from build123d import *

# Parameters (mm, degrees)
SKETCH_W     = 80
SKETCH_H     = 26
PAD_DEPTH    = 2
SKETCH001_W  = 73.5
SKETCH001_H  = 21.5
PAD001_DEPTH = 2
SKETCH002_W  = 1.5
SKETCH002_H  = 20
POCKET_DEPTH = 5
CHAMFER_SIZE = 1.5


with BuildPart() as part:
    # Sketch → Pad (new body)
    with BuildSketch(Plane.XY):
        Rectangle(SKETCH_W, SKETCH_H)
    extrude(amount=PAD_DEPTH)

    # Sketch001 (on Face6 of Pad) → Pad001 (join)
    with BuildSketch(Plane.XY.offset(2)):
        Rectangle(SKETCH001_W, SKETCH001_H)
    extrude(amount=PAD001_DEPTH)

    # Sketch002 (on Face11 of Pad001) → Pocket (cut)
    with BuildSketch(Plane.XY.offset(4)):
        with Locations((1.5, 0)):
            Rectangle(SKETCH002_W, SKETCH002_H)
        with Locations((4.5, 0)):
            Rectangle(SKETCH002_W, SKETCH002_H)
        with Locations((7.5, 0)):
            Rectangle(SKETCH002_W, SKETCH002_H)
        with Locations((10.5, 0)):
            Rectangle(SKETCH002_W, SKETCH002_H)
        with Locations((13.5, 0)):
            Rectangle(SKETCH002_W, SKETCH002_H)
        with Locations((16.5, 0)):
            Rectangle(SKETCH002_W, SKETCH002_H)
        with Locations((19.5, 0)):
            Rectangle(SKETCH002_W, SKETCH002_H)
        with Locations((22.5, 0)):
            Rectangle(SKETCH002_W, SKETCH002_H)
        with Locations((25.5, 0)):
            Rectangle(SKETCH002_W, SKETCH002_H)
        with Locations((28.5, 0)):
            Rectangle(SKETCH002_W, SKETCH002_H)
        with Locations((31.5, 0)):
            Rectangle(SKETCH002_W, SKETCH002_H)
        with Locations((34.5, 0)):
            Rectangle(SKETCH002_W, SKETCH002_H)
        with Locations((-1.5, 0)):
            Rectangle(SKETCH002_W, SKETCH002_H)
        with Locations((-4.5, 0)):
            Rectangle(SKETCH002_W, SKETCH002_H)
        with Locations((-7.5, 0)):
            Rectangle(SKETCH002_W, SKETCH002_H)
        with Locations((-10.5, 0)):
            Rectangle(SKETCH002_W, SKETCH002_H)
        with Locations((-13.5, 0)):
            Rectangle(SKETCH002_W, SKETCH002_H)
        with Locations((-16.5, 0)):
            Rectangle(SKETCH002_W, SKETCH002_H)
        with Locations((-19.5, 0)):
            Rectangle(SKETCH002_W, SKETCH002_H)
        with Locations((-22.5, 0)):
            Rectangle(SKETCH002_W, SKETCH002_H)
        with Locations((-25.5, 0)):
            Rectangle(SKETCH002_W, SKETCH002_H)
        with Locations((-28.5, 0)):
            Rectangle(SKETCH002_W, SKETCH002_H)
        with Locations((-31.5, 0)):
            Rectangle(SKETCH002_W, SKETCH002_H)
        with Locations((-34.5, 0)):
            Rectangle(SKETCH002_W, SKETCH002_H)
    extrude(amount=-POCKET_DEPTH, mode=Mode.SUBTRACT)

    # Chamfer
    chamfer_edges = [part.edges().sort_by_distance(p)[0] for p in [
        (0, -13, 0),
        (40, 0, 0),
        (0, 13, 0),
        (-40, 0, 0),
    ]]
    chamfer(chamfer_edges, length=CHAMFER_SIZE)


solid = part.part
Model file for the job. Use its own axes, mm. Give positions to 0.01 mm unless a question says otherwise; leave off trailing zeros. Loops run counter-clockwise (first coordinate to the right, second up) from the corner with the lowest first, then second, coordinate; pieces in that order, holes last.
1) Saw through at B-B (y = 8.25). Count the separate pieces of the cut face and the enclosed holes in it, plus the area to 3 significant figures.
2) Saw through at A-A (x = -19.5). Write the cut outline in (y, z).
3) Pull direction Y, two halves, no side cores. Call faces 1 (the flat face through (36.75, 0, 3)), 2 (the flat face through (18.75, 0, 2)), 3 (the flat face through (-0.6, -12.2, 0.7)): +Y half, -Y half, draft (parallel to the pull), parting line (faces both ways), or undercut.
4) Wall check: line 1 (Y direction, x = 13.5, z = 1.7); line 2 (Y direction, x = 25, z = 3); line 3 (Y direction, x = -15, z = 3.1). Give the ranges that are in metal, low to high.
5) Flat gauge pins, fed straight in: pin 1 Ø0.8 at (x, z) = (-13.5, 3) entering from -Y; pin 2 Ø6 at (x, y) = (-18, -2.5) entering from -Z. Where does each tip first touch, or does it go through?
Answer block:
1. separate pieces: 25
1. enclosed holes: 0
1. area: 161 mm2
2. outline: (-13, 1.5) - (-11.5, 0) - (-10, 0) - (-10, 4) - (-10.75, 4) - (-10.75, 2) - (-13, 2) - close; (10, 0) - (11.5, 0) - (13, 1.5) - (13, 2) - (10.75, 2) - (10.75, 4) - (10, 4) - close
3. face 1: draft
3. face 2: undercut
3. face 3: -Y half
4. line 1: y = -13 to -10, 10 to 13
4. line 2: y = -10.75 to -10, 10 to 10.75
4. line 3: y = -10.75 to 10.75
5. pin 1: stops at y = -10.75
5. pin 2: stops at z = 0
